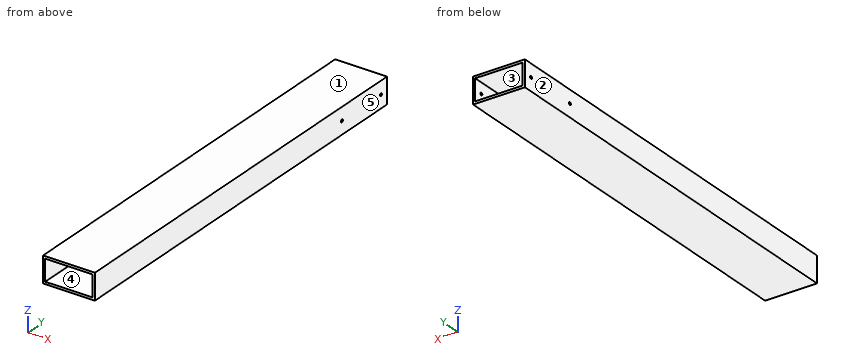
```python
from build123d import *

# Parameters (mm, degrees)
SKETCH1_W           = 38.1
SKETCH1_H           = 19.05
SKETCH1_W_2         = 34.798
SKETCH1_H_2         = 15.748
BOSS_EXTRUDE1_DEPTH = 304.8
SKETCH2_R           = 1.016
CUT_EXTRUDE1_DEPTH  = 39.1


with BuildPart() as part:
    # Sketch1 → Boss-Extrude1 (new body)
    with BuildSketch(Plane(origin=(0, 0, 0), x_dir=(1, 0, 0), z_dir=(0, 1, 0))):
        Rectangle(SKETCH1_W, SKETCH1_H)
        Rectangle(SKETCH1_W_2, SKETCH1_H_2, mode=Mode.SUBTRACT)
    extrude(amount=BOSS_EXTRUDE1_DEPTH)

    # Sketch2 → Cut-Extrude1 (cut, through all)
    with BuildSketch(Plane(origin=(19.05, 0, 0), x_dir=(0, 0, -1), z_dir=(1, 0, 0))):
        with Locations((0, 298.45)):
            Circle(SKETCH2_R)
        with Locations((0, 257.81)):
            Circle(SKETCH2_R)
    extrude(amount=-CUT_EXTRUDE1_DEPTH, mode=Mode.SUBTRACT)


solid = part.part
```
Part model, mm, in its own coordinate system. Face numbers are marked on the shaded views. A direction names the side the tool comes from. Round coordinates to 2 decimals unless told otherwise and drop trailing zeros. Write each loop counter-clockwise with the first axis right and the second up, starting at its lowest first coordinate (ties: lowest second). Pieces come first, ordered by that corner, then holes. Notation, with made-up numbers: M 21,-12.75 L 54,-12.75 A4 cw 54,-6.75 Z; hole C 35,58 d4. An arc over 180 degrees is marked long. Answer as CSV lines item,"result". Start each with the question number.
1) Which spindle directions (+Z, -Z, +X, -X, +Y, -Y) get a long thin tool onto all of the face, cutting with end or side? Do the marked faces 4 and 5. Say none if no direction does.
2) Band-saw the part on B-B (x = 2). List the corners of the cut face in (y, z) (3 decimals).
3) Drop flat-ended pins along their axis: pin 1 (2.5 mm diameter, centred on y = 298.45, z = 0, fed in from +X); pin 2 (1.8 mm diameter, centred on y = 257.81, z = 0, fed in from +X). Give the stop position or say it passes through.
4) Band-saw the part on C-C (y = 134.5). List the corners of the cut face in (x, z) (3 decimals), then the cut area to 3 significant figures.
5) Band-saw the part on A-A (z = 4.25). List the corners of the cut face in (x, y), then the cut area to 3 significant figures.
6) Mould opens along Z. For the marked faces 1, 2 and 3 say: +Z half, -Z half, draft (parallel to the pull), parting line (faces both ways), or undercut.
7) Drill centre lines: L1, parallel to Y at x = 18.1, z = 0; L2, parallel to X at y = 102.5, z = -7; L3, parallel to Z at x = -6, y = 78 (3 decimals). Where is each one in solid material? Low to high.
Worked out:
1,face 4,"+Y, -Y"
1,face 5,"+Z, -Z, +X, +Y, -Y"
2,outline,"M 0,-9.525 L 304.8,-9.525 L 304.8,-7.874 L 0,-7.874 Z; M 0,7.874 L 304.8,7.874 L 304.8,9.525 L 0,9.525 Z"
3,pin 1,"x = 19.05"
3,pin 2,"through"
4,outline,"M -19.05,-9.525 L 19.05,-9.525 L 19.05,9.525 L -19.05,9.525 Z; hole M -17.399,-7.874 L 17.399,-7.874 L 17.399,7.874 L -17.399,7.874 Z"
4,area,"178 mm²"
5,outline,"M -19.05,0 L -17.4,0 L -17.4,304.8 L -19.05,304.8 Z; M 17.4,0 L 19.05,0 L 19.05,304.8 L 17.4,304.8 Z"
5,area,"1,010 mm²"
6,face 1,"+Z half"
6,face 2,"draft"
6,face 3,"undercut"
7,L1,"0 to 256.79, 258.83 to 297.43, 299.47 to 304.8"
7,L2,"-19.05 to -17.4, 17.4 to 19.05"
7,L3,"-9.525 to -7.874, 7.874 to 9.525"
